Design review of the part built by this model. Coordinates are the model's own, in mm. Face numbers are marked on the shaded views. A direction names the side the tool comes from. Round coordinates to 2 decimals unless told otherwise and drop trailing zeros. Loops run counter-clockwise (first coordinate to the right, second up) from the corner with the lowest first, then second, coordinate; pieces in that order, holes last. Notation, with made-up numbers: M 89,75.5 L 142,75.5 A14 ccw 142,80.5 Z; hole C 62.5,-25 d6. An arc over 180 degrees is marked long. Use a Markdown table: item, result.
Autodesk Inventor part; units mm, degrees
ref_plane "YZ Plane" through (0, 0, 0) normal (1, 0, 0) x (0, 1, 0)
ref_plane "XZ Plane" through (0, 0, 0) normal (0, 1, 0) x (-1, 0, 0)
ref_plane "XY Plane" through (0, 0, 0) normal (0, 0, 1) x (1, 0, 0)
sketch "스케치1" plane through (0, 0, 0) normal (0, 0, 1) x (1, 0, 0)
  line L0 (0, 0) -> (150, 0)
  line L1 (150, 0) -> (150, -145)
  line L2 (150, -145) -> (0, -145)
  line L3 (0, -145) -> (0, 0)
  line L4 (0, -20) -> (150, -20)
  line L5 (0, -125) -> (150, -125)
  line L6 (150, -135) -> (0, -135)
  line L7 (150, -10) -> (0, -10)
  circle A0 centre (21.5, -99.25) radius 2.5
  line L8 (75, -145) -> (75, -139.9922)
  circle A1 centre (128.5, -99.25) radius 2.5
  circle A2 centre (5, -5) radius 1.5
  circle A3 centre (145, -5) radius 1.5
  circle A4 centre (5, -140) radius 1.5
  circle A5 centre (145, -140) radius 1.5
  dimension "d0" = 150
  dimension "d1" = 145
  dimension "d2" = 20
  dimension "d3" = 20
  dimension "d8" = 10
  dimension "d9" = 10
  dimension "d21" = 45.75
  dimension "d22" = 21.5
  dimension "d23" = 5
  dimension "d24" = 3
  dimension "d25" = 5
  dimension "d26" = 5
  dimension "d27" = 5
  dimension "d28" = 5
  dimension "d29" = 5
extrude "돌출1" add sketch "스케치1" along normal blind 10 contours L7 L1 L4 L3 | L4 L1 L5 L3 | L5 L1 L6 L3
extrude "돌출2" add sketch "스케치1" against normal blind 50 contours L0 L1 L7 L3 | L7 L1 L4 L3 | L5 L1 L6 L3 | L6 L1 L2 L3 | A2 | A3 | A4 | A5
extrude "돌출3" cut sketch "스케치1" against normal blind 40 contours L0 L1 L7 L3 | L6 L1 L2 L3 | A2 | A3 | A4 | A5
sketch "스케치2" plane through (0, 0, 10) normal (0, 0, 1) x (1, 0, 0)
  circle A0 centre (20, -30) radius 2.5
  circle A1 centre (130, -30) radius 2.5
  line L0 (150, -135) -> (150, -10)
  line L1 (0, -10) -> (0, -135)
  line L2 (0, 0) -> (150, 0)
  circle A2 centre (20, -50) radius 2.5
  circle A3 centre (130, -50) radius 2.5
  circle A4 centre (75, -72.5) radius 25
  point P0 (0, -72.5)
  point P1 (0, -72.5)
  point P2 (75, 0)
  dimension "d14" = 20
  dimension "d15" = 20
  dimension "d16" = 5
  dimension "d17" = 30
  dimension "d18" = 5
  dimension "d19" = 20
  dimension "d20" = 50
extrude "돌출4" cut sketch "스케치2" against normal through all
extrude "돌출5" cut sketch "스케치1" against normal through all contours A2 | A3 | A4 | A5
sketch "스케치3" plane through (150, -135, 10) normal (1, 0, 0) x (0, 0, -1)
  circle A0 centre (55, 120) radius 1.5
  circle A1 centre (5, 120) radius 1.5
  circle A2 centre (5, 5) radius 1.5
  circle A3 centre (55, 5) radius 1.5
  line L0 (50, -10) -> (60, -10)
  line L1 (0, 0) -> (0, 125)
  line L2 (10, 10) -> (10, 115)
  line L3 (0, 0) -> (50, 0)
  line L4 (10, 10) -> (60, 10)
  point P0 (10, 135)
  point P1 (55, -10)
  dimension "d32" = 3
  dimension "d33" = 10
  dimension "d34" = 5
  dimension "d35" = 10
  dimension "d36" = 5
  dimension "d37" = 5
extrude "돌출6" cut sketch "스케치3" against normal through all
equation "\"d8\" = 0.5 * d2"
equation "\"d9\" = d8"
equation "\"d25\" = 0.5 * d9"
equation "\"d26\" = d25"
equation "\"d27\" = d25"
equation "\"d28\" = d25"
equation "\"d29\" = d27"
equation "\"d34\" = 0.5 * d33"
equation "\"d36\" = 0.5 * d35"
equation "\"d37\" = 0.5 * d35"
properties part number "WheelCorver_3D 인쇄"
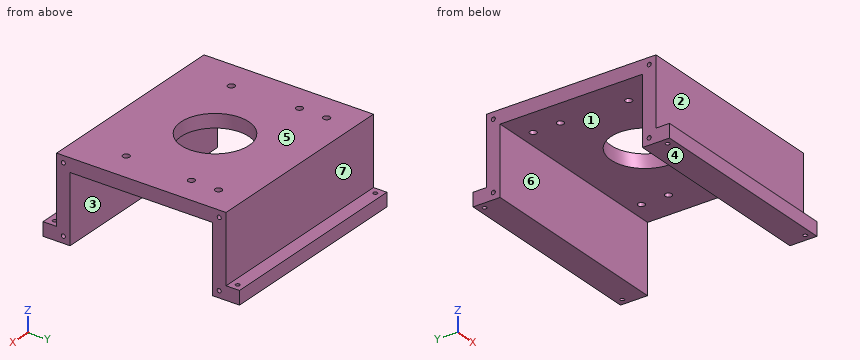
1. Machinability: for the marked faces 5, 6 and 7, which of the approach directions +Z, -Z, +X, -X, +Y, -Y give a long, thin tool a straight path to every point of the face, cutting with its end or side? Answer none if there is none.
Check values:
| item | result |
|---|---|
| face 5 | +Z, +X, -X, +Y, -Y |
| face 6 | -Z, +X, -X |
| face 7 | +Z, +X, -X, +Y |
2. Insertion check: pin 1 (1.8 mm diameter, centred on y = -15, z = -45, fed in from +X); pin 2 (6 mm diameter, centred on x = 130, y = -30, fed in from -Z); pin 3 (8 mm diameter, centred on x = 61.5, y = -140.5, fed in from +Z); pin 4 (1 mm diameter, centred on x = 39.5, z = -24.5, fed in from +Y). Each pin has a flat end and moves straight along its axis. Give the tip position at first contact, or say it passes through.
Check values:
| item | result |
|---|---|
| pin 1 | passes through |
| pin 2 | stops at z = 0 |
| pin 3 | stops at z = -40 |
| pin 4 | stops at y = -10 |
3. Take a section at A-A on x = 116. Give the boundary of the cut face in (y, z).
Check values:
| item | result |
|---|---|
| outline | M -145,-50 L -125,-50 L -125,0 L -20,0 L -20,-50 L 0,-50 L 0,-40 L -10,-40 L -10,10 L -135,10 L -135,-40 L -145,-40 Z; hole C -130,-45 d3; hole C -130,5 d3; hole C -15,-45 d3; hole C -15,5 d3 |
4. Take a section at D-D on x = 93. Give the boundary of the cut face in (y, z).
Check values:
| item | result |
|---|---|
| outline | M -145,-50 L -125,-50 L -125,0 L -89.85,0 L -89.85,10 L -135,10 L -135,-40 L -145,-40 Z; M -55.15,0 L -20,0 L -20,-50 L 0,-50 L 0,-40 L -10,-40 L -10,10 L -55.15,10 Z; hole C -130,-45 d3; hole C -130,5 d3; hole C -15,-45 d3; hole C -15,5 d3 |
5. Wall thickness on line 1 along Y through (x, z) = (145, -45); line 2 along Y through (x, z) = (71.5, -17); line 3 along Z through (x, y) = (69, -130): over which ranges is each line inside the solid? List them lowest first. Write a range as from..to.
Check values:
| item | result |
|---|---|
| line 1 | y = -145..-141.5, -138.5..-131.5, -128.5..-125, -20..-16.5, -13.5..-6.5, -3.5..0 |
| line 2 | y = -135..-125, -20..-10 |
| line 3 | z = -50..-46.5, -43.5..3.5, 6.5..10 |
6. Take a section at B-B on y = -72.5. Give the boundary of the cut face in (x, z).
Check values:
| item | result |
|---|---|
| outline | M 0,0 L 50,0 L 50,10 L 0,10 Z; M 100,0 L 150,0 L 150,10 L 100,10 Z |
7. Take a section at C-C on z = -3. Give the boundary of the cut face in (x, y).
Check values:
| item | result |
|---|---|
| outline | M 0,-135 L 150,-135 L 150,-125 L 0,-125 Z; M 0,-20 L 150,-20 L 150,-10 L 0,-10 Z |
8. The part is to be moulded in two halves that separate along Y. For the marked faces 1, 2, 3 and 4, say which applies: pulls with the +Y half, pulls with the -Y half, needs draft (parallel to the pull), parting line crosses it, or undercut.
Check values:
| item | result |
|---|---|
| face 1 | undercut |
| face 2 | pulls with the -Y half |
| face 3 | undercut |
| face 4 | needs draft |
